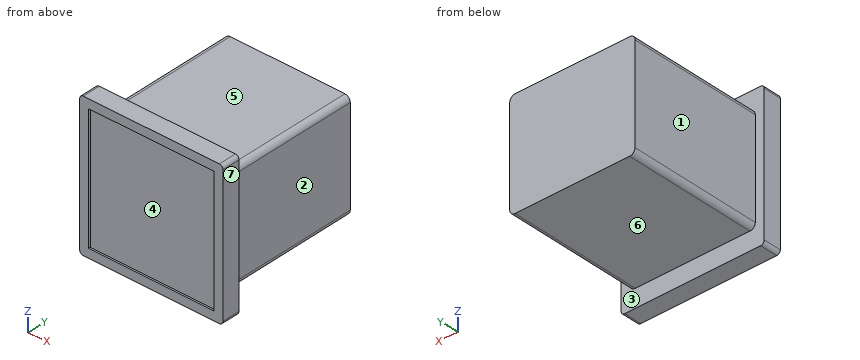
from build123d import *

# Parameters (mm, degrees)
F0_W     = 80
F0_H     = 80
F1_DEPTH = 10
F2_R     = 2
F3_W     = 70
F3_H     = 70
F4_DEPTH = 1
F5_W     = 70
F5_H     = 60
F6_DEPTH = 75
F7_R     = 3


with BuildPart() as f1:
    # F0 (on Front) → F1 (new body)
    with BuildSketch(Plane.XZ):
        Rectangle(F0_W, F0_H)
    extrude(amount=F1_DEPTH)

    # F2
    f2_edges = [f1.edges().sort_by_distance(p)[0] for p in [
        (-40, -5, 40),
        (40, -5, 40),
        (40, -5, -40),
        (-40, -5, -40),
    ]]
    fillet(f2_edges, radius=F2_R)

    # F3 (on face) → F4 (cut)
    with BuildSketch(Plane.XZ.offset(10)):
        Rectangle(F3_W, F3_H)
    extrude(amount=-F4_DEPTH, mode=Mode.SUBTRACT)

    # F5 (on face) → F6 (join)
    with BuildSketch(Plane(origin=(0, 0, 0), x_dir=(-1, 0, 0), z_dir=(0, 1, 0))):
        Rectangle(F5_W, F5_H)
    extrude(amount=F6_DEPTH)

    # F7
    f7_edges = [f1.edges().sort_by_distance(p)[0] for p in [
        (35, 37.5, 30),
        (-35, 37.5, 30),
        (35, 37.5, -30),
        (-35, 37.5, -30),
    ]]
    fillet(f7_edges, radius=F7_R)


solid = f1.part
The model under review builds one solid part; all positions refer to its coordinate system, in mm. Face numbers are marked on the shaded views. A direction names the side the tool comes from. Coordinates: 2 decimals unless noted, no trailing zeros. Write each loop counter-clockwise with the first axis right and the second up, starting at its lowest first coordinate (ties: lowest second). Pieces come first, ordered by that corner, then holes. Notation, with made-up numbers: (87, 64) - (110, 64) arc R21 ccw to (110, 78) - close; hole circle Ø9 at (-23, 14). An arc over 180 degrees is marked (long way). Answer as CSV lines item,"result".
(1) We need section A-A (x = 13.5). Give the boundary of the cut face in (y, z).
Data:
outline,"(-10, -40) - (0, -40) - (0, -30) - (75, -30) - (75, 30) - (0, 30) - (0, 40) - (-10, 40) - (-10, 35) - (-9, 35) - (-9, -35) - (-10, -35) - close"
(2) Mouldability with a two-part tool opening along Z and no side actions: class the marked faces 4, 5, 6 and 7 as pulls with the +Z half, pulls with the -Z half, needs draft (parallel to the pull), parting line crosses it, or undercut.
Data:
face 4,"undercut"
face 5,"pulls with the +Z half"
face 6,"pulls with the -Z half"
face 7,"needs draft"
(3) We need section C-C (z = -4.5). Give the boundary of the cut face in (x, y).
Data:
outline,"(-40, -10) - (-35, -10) - (-35, -9) - (35, -9) - (35, -10) - (40, -10) - (40, 0) - (35, 0) - (35, 75) - (-35, 75) - (-35, 0) - (-40, 0) - close"
(4) Clearance check with flat-ended pins moving along their axes: pin 1 Ø1 at (x, y) = (-29, 45.5) entering from -Z; pin 2 Ø6 at (x, z) = (7, -24.5) entering from -Y; pin 3 Ø12 at (x, y) = (6, 39) entering from +Z. State where each tip first meets the part, or that it passes through.
Data:
pin 1,"stops at z = -30"
pin 2,"stops at y = -9"
pin 3,"stops at z = 30"
(5) For line 1 along X through (y, z) = (1.5, -7); line 2 along Z through (x, y) = (-22, 5); line 3 along Y through (x, z) = (-5.5, -37), list the stretches that pass through material, from the lowest coordinate up. Write a range as [from, to].
Data:
line 1,"x = [-35, 35]"
line 2,"z = [-30, 30]"
line 3,"y = [-10, 0]"
(6) Tool access review of the marked faces 1, 2 and 3: name each direction out of +Z, -Z, +X, -X, +Y, -Y from which nothing blocks a thin tool from reaching the whole face with its end or side.
Data:
face 1,"+Z, -Z, -X, +Y"
face 2,"+Z, -Z, +X, +Y"
face 3,"+Y"
(7) We need section B-B (y = 10). Give the boundary of the cut face in (x, z).
Data:
outline,"(-35, -27) arc R3 ccw to (-32, -30) - (32, -30) arc R3 ccw to (35, -27) - (35, 27) arc R3 ccw to (32, 30) - (-32, 30) arc R3 ccw to (-35, 27) - close"
